from build123d import *

# Parameters (mm, degrees)
F1_DEPTH = 100
F2_DEPTH = 25
F4_DEPTH = 75
F5_DEPTH = 75


with BuildPart() as f1:
    # F0 (on Front) → F1 (new body)
    with BuildSketch(Plane.XZ):
        Polygon((75, 0), (25, 20), (-25, 20), (-75, 0), align=None)
    extrude(amount=F1_DEPTH)

    # F1_face (on face) → F2 (join)
    with BuildSketch(Plane(origin=(0, -100, 8.333333), x_dir=(1, 0, 0), z_dir=(0, -1, 0))):
        Polygon((75, -8.333333), (25, 11.666667), (-25, 11.666667), (-75, -8.333333), align=None)
    extrude(amount=F2_DEPTH)

    # F3 (on Right) → F4 (join)
    with BuildSketch(Plane.YZ):
        Polygon((-124.444783, 0), (-100.156426, 0), (-100.156426, 19.705653), align=None)
    extrude(amount=F4_DEPTH)

    # F3 (on Right) → F5 (join)
    with BuildSketch(Plane.YZ):
        Polygon((-124.444783, 0), (-100.156426, 0), (-100.156426, 19.705653), align=None)
    extrude(amount=-F5_DEPTH)


solid = f1.part
Source: CAD feature listing. Evaluate the final solid. Frame: model axes, mm. A direction names the side the tool comes from. Give positions to 0.01 mm unless a question says otherwise; leave off trailing zeros. Write each loop counter-clockwise with the first axis right and the second up, starting at its lowest first coordinate (ties: lowest second). Pieces come first, ordered by that corner, then holes. Notation, with made-up numbers: M -2,-33 L 2,-33 A18 cw 2,0 Z; hole C 82,16 d3. An arc over 180 degrees is marked long. Answer as a JSON object with one key per item and string values.
Q1. Cut plane D-D, the plane x = 42.5. Return the cut outline in (y, z), then the cut area to 3 significant figures.
Geometry check:
{"outline": "M -125,0 L 0,0 L 0,13 L -100.16,13 L -100.16,19.71 L -108.42,13 L -125,13 Z", "area": "1,650 mm^2"}
Q2. Ray query, line 1 along Z through (x, y) = (36, -94); line 2 along Z through (x, y) = (28, -87.5); line 3 along Y through (x, z) = (-64, 7). Return the intervals inside material, ascending.
Geometry check:
{"line 1": "z = 0 to 15.6", "line 2": "z = 0 to 18.8", "line 3": "y = -115.82 to -100.16"}
Q3. Access query for faces 1 (the face through (61, -100.156, 14)), 2 (the face through (-60.97, -106.73, 14.37)), 3 (the face through (60.97, -106.73, 14.37)). Directions: +Z, -Z, +X, -X, +Y, -Y. A direction counts if a zero-diameter tool reaches every point of the face in a straight line with its end or side. Return the directions, or none.
Geometry check:
{"face 1": "+Z, +X, +Y", "face 2": "+Z, -X, -Y", "face 3": "+Z, +X, -Y"}
Q4. Cut plane C-C, the plane z = 1.75. Return the cut outline in (x, y) (3 decimals), then the cut area to 3 significant figures.
Geometry check:
{"outline": "M -75,-122.288 L -70.625,-122.288 L -70.625,-125 L 70.625,-125 L 70.625,-122.288 L 75,-122.288 L 75,-100.156 L 70.625,-100.156 L 70.625,0 L -70.625,0 L -70.625,-100.156 L -75,-100.156 Z", "area": "17,800 mm^2"}
Q5. Cut plane A-A, the plane x = -59. Return the cut outline in (y, z).
Geometry check:
{"outline": "M -125,0 L 0,0 L 0,6.4 L -100.16,6.4 L -100.16,19.71 L -116.56,6.4 L -125,6.4 Z"}
Q6. Cut plane B-B, the plane y = -88.5. Return the cut outline in (x, z).
Geometry check:
{"outline": "M -75,0 L 75,0 L 25,20 L -25,20 Z"}
Q7. Contact query for flat-ended pins moving along their axis: P1, Ø10, axis at x = -50, y = -91, coming from the -Z side; P2, Ø10, axis at x = -61.5, z = 13.5, coming from the +Y side. Output: stop coordinate, or through.
Geometry check:
{"P1": "stops at z = 0", "P2": "stops at y = -100.16"}
